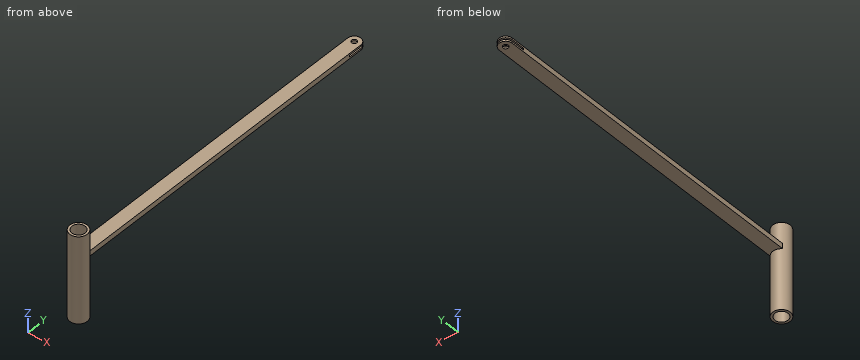
from build123d import *

# Parameters (mm, degrees)
SKETCH_1_R           = 10
SKETCH_1_R_2         = 7.5
EXTRUDE_1_DEPTH      = 50
EXTRUDE_2_REACH      = 399.792
EXTRUDE_2_END_RADIUS = 10
SKETCH_2_W           = 15
SKETCH_2_H           = 6
FILLET_1_R           = 7.5
SKETCH_3_R           = 3
CUT_EXTRUDE_1_DEPTH  = 10
SKETCH_4_W           = 2
SKETCH_4_H           = 23
CUT_EXTRUDE_2_DEPTH  = 20


with BuildPart() as part:
    # 草图1 → 凸台-拉伸1 (new, symmetric)
    with BuildSketch(Plane.XY):
        Circle(SKETCH_1_R)
        Circle(SKETCH_1_R_2, mode=Mode.SUBTRACT)
    extrude(amount=EXTRUDE_1_DEPTH, both=True)

    # 凸台-拉伸2: up to this cylinder (the profile starts outside it)
    extrude_2_end = Plane(origin=(0, 0, 22.779793), z_dir=(0, 0, -1)) * Cylinder(EXTRUDE_2_END_RADIUS, 820.584, mode=Mode.PRIVATE)
    # 草图2 → 凸台-拉伸2 (add, up to the surface)
    with BuildSketch(Plane(origin=(0, 384.51, 0), x_dir=(1, 0, 0), z_dir=(0, 1, 0)), mode=Mode.PRIVATE) as extrude_2_sk1:
        with Locations((0.280971345, -22.779792891)):
            Rectangle(SKETCH_2_W, SKETCH_2_H)
    extrude_2_tool1 = extrude(extrude_2_sk1.sketch, amount=-EXTRUDE_2_REACH, mode=Mode.PRIVATE) - extrude_2_end
    add(extrude_2_tool1.solids().sort_by_distance((0.280971, 384.51, 22.779793))[0])

    # 圆角1
    fillet_1_edges = [part.edges().sort_by_distance(p)[0] for p in [
        (7.780971345, 384.51, 22.779792891),
        (-7.219028655, 384.51, 22.779792891),
    ]]
    fillet(fillet_1_edges, radius=FILLET_1_R - 0.0001)  # a hair under: the kernel refuses the full size

    # 草图3 → 切除-拉伸1 (cut)
    with BuildSketch(Plane(origin=(0, 0, 19.779792891), x_dir=(-1, 0, 0), z_dir=(0, 0, -1))):
        with Locations((-0.280971345, 377.01)):
            Circle(SKETCH_3_R)
    extrude(amount=-CUT_EXTRUDE_1_DEPTH, mode=Mode.SUBTRACT)

    # 草图4 → 切除-拉伸2 (cut)
    with BuildSketch(Plane.ZY.offset(7.219028655)):
        with Locations((22.779792891, 373.01)):
            Rectangle(SKETCH_4_W, SKETCH_4_H)
    extrude(amount=-CUT_EXTRUDE_2_DEPTH, mode=Mode.SUBTRACT)


solid = part.part
CAD build for the part. Positions are in the model's coordinates, mm. Round coordinates to 2 decimals unless told otherwise and drop trailing zeros. Loops run counter-clockwise (first coordinate to the right, second up) from the corner with the lowest first, then second, coordinate; pieces in that order, holes last.
(1) Cut at B-B (z = 5.5). Give the cut face in (x, y).
(2) Drop flat-ended pins along their axis: pin 1 (1 mm diameter, centred on x = 4, z = 34.5, fed in from +Y); pin 2 (3 mm diameter, centred on y = 117.5, z = 22.5, fed in from -X); pin 3 (4.5 mm diameter, centred on x = -1.5, y = 368.5, fed in from -Z); pin 4 (12 mm diameter, centred on x = 0, y = 0, fed in from +Z). Give the stop position or say it passes through.
(3) Cut at A-A (y = 0). Give the cut face in (x, z), plus the area to 3 significant figures.
(4) Wall check: line 1 along Y through (x, z) = (1, 19); line 2 along Y through (x, z) = (0, -7); line 3 along X through (y, z) = (377, 25). Give the ranges that are in metal, low to high.
Findings below:
1. outline: circle Ø20 at (0, 0); hole circle Ø15 at (0, 0)
2. pin 1: stops at y = 9.37
2. pin 2: stops at x = -7.22
2. pin 3: stops at z = 19.78
2. pin 4: passes through
3. outline: (-10, -50) - (-7.5, -50) - (-7.5, 50) - (-10, 50) - close; (7.5, -50) - (10, -50) - (10, 50) - (7.5, 50) - close
3. area: 500 mm2
4. line 1: y = -9.95 to -7.43, 7.43 to 9.95
4. line 2: y = -10 to -7.5, 7.5 to 10
4. line 3: x = -7.22 to -2.72, 3.28 to 7.78
